Could you check a few things on this model? Use its own coordinates, in mm. A direction names the side the tool comes from. Coordinates: 2 decimals unless noted, no trailing zeros. Order: outer loops, then holes, each group sorted by start corner. A loop starts at its lowest first (then second) coordinate and runs counter-clockwise, first axis right, second up. Notation, with made-up numbers: (32, -9) - (38, -9) arc R6 ccw to (38, -2) - close; hole circle Ø9 at (-24, 39.5). An arc over 180 degrees is marked (long way). Answer as CSV lines item,"result". Start each with the question number.
1. I want a section at A-A, the plane x = 33. List the corners of the cut face in (y, z) for me, and give its area (3 significant figures).
2. I want a section at D-D, the plane y = -14.5. Count the separate pieces of the cut face and the enclosed holes in it, and give its area (3 significant figures).
3. I want a section at B-B, the plane z = -8.5. List the corners of the cut face in (x, y) for me.
4. I need wall thicknesses on probe 1 along X at (y, z) = (-12.7, -10); probe 2 along Y at (x, z) = (38.1, -8); probe 3 along X at (y, z) = (-14.75, -16.5). Which ranges of each line are inside material? Lowest first, please.
5. For faces 1 (the face through (25, -10, -2.108)), 2 (the face through (23, 0, -1)), 3 (the face through (48.692, -10, -13)), which set-ups out of +Z, -Z, +X, -X, +Y, -Y let a thin tool reach every point of the face, with its end or its side?
6. I want a section at C-C, the plane y = -3. List the corners of the cut face in (x, z) for me, and give its area (3 significant figures).
7. For pin 1 (6 mm diameter, centred on y = -19.5, z = -7, fed in from +X); pin 2 (5 mm diameter, centred on x = 44.5, y = -17.5, fed in from -Z); pin 3 (6 mm diameter, centred on x = 12.7, y = -12.7, fed in from +Z), each with a flat end and sliding along its axis, tell me the tip position at first contact or that it passes through.
8. Thinking about a two-plate mould opening in Y: for faces 4 (the face through (35.754, -13.673, -19.247)), 5 (the face through (25, -25.4, -13)), 6 (the face through (11.33, -10.56, -6.3)), 7 (the face through (25, -10, -23.292)), which applies, released by +Y, released by -Y, zero draft, split by the parting line, or undercut?
from build123d import *

# Parameters (mm, degrees)
SKETCH2_W           = 50.8
SKETCH2_H           = 25.4
BOSS_EXTRUDE2_DEPTH = 1.999996
SKETCH2_4_W         = 46.5836
SKETCH2_4_H         = 21.1836
BOSS_EXTRUDE3_DEPTH = 25.4
FILLET3_R           = 0.810638298
SKETCH3_R           = 2.54
CUT_EXTRUDE1_DEPTH  = 49.6918
SKETCH4_R           = 2.54
CUT_EXTRUDE2_DEPTH  = 24.2918


with BuildPart() as part:
    # Sketch2 → Boss-Extrude2 (new body)
    with BuildSketch(Plane(origin=(0, 0, 0), x_dir=(1, 0, 0), z_dir=(0, 1, 0))):
        with Locations((25.4, 12.7)):
            Rectangle(SKETCH2_W, SKETCH2_H)
    extrude(amount=BOSS_EXTRUDE2_DEPTH)

    # Sketch2<4> → Boss-Extrude3 (add)
    with BuildSketch(Plane(origin=(0, 0, 0), x_dir=(1, 0, 0), z_dir=(0, 1, 0))):
        with Locations((25.4, 12.7)):
            Rectangle(SKETCH2_4_W, SKETCH2_4_H)
    extrude(amount=-BOSS_EXTRUDE3_DEPTH)

    # Fillet3
    fillet3_edges = [part.edges().sort_by_distance(p)[0] for p in [
        (2.1082, -12.7, -2.1082),
        (2.1082, -12.7, -23.2918),
        (48.6918, -12.7, -23.2918),
        (48.6918, -12.7, -2.1082),
    ]]
    fillet(fillet3_edges, radius=FILLET3_R)

    # Sketch3 → Cut-Extrude1 (cut, through all)
    with BuildSketch(Plane(origin=(48.6918, 0, 0), x_dir=(0, 0, -1), z_dir=(1, 0, 0))):
        with Locations((12.7, -12.7)):
            Circle(SKETCH3_R)
    extrude(amount=-CUT_EXTRUDE1_DEPTH, mode=Mode.SUBTRACT)

    # Sketch4 → Cut-Extrude2 (cut, through all)
    with BuildSketch(Plane(origin=(0, 0, -23.2918), x_dir=(-1, 0, 0), z_dir=(0, 0, -1))):
        with Locations((-25.4, -12.7)):
            Circle(SKETCH4_R)
        with Locations((-38.1, -12.7)):
            Circle(SKETCH4_R)
        with Locations((-12.7, -12.7)):
            Circle(SKETCH4_R)
    extrude(amount=-CUT_EXTRUDE2_DEPTH, mode=Mode.SUBTRACT)


solid = part.part
Solved:
1,outline,"(-25.4, -23.29) - (0, -23.29) - (0, -25.4) - (2, -25.4) - (2, 0) - (0, 0) - (0, -2.11) - (-25.4, -2.11) - close; hole circle Ø5.08 at (-12.7, -12.7)"
1,area,"569 mm2"
2,separate pieces,"8"
2,enclosed holes,"0"
2,area,"630 mm2"
3,outline,"(0, 0) - (2.11, 0) - (2.11, -25.4) - (48.69, -25.4) - (48.69, 0) - (50.8, 0) - (50.8, 2) - (0, 2) - close; hole circle Ø5.08 at (12.7, -12.7); hole circle Ø5.08 at (25.4, -12.7); hole circle Ø5.08 at (38.1, -12.7)"
4,probe 1,"x = 2.11 to 10.16, 15.24 to 22.86, 27.94 to 35.56, 40.64 to 48.69"
4,probe 2,"y = -25.4 to -15.24, -10.16 to 2"
4,probe 3,"x = 2.11 to 11.2, 14.2 to 23.9, 26.9 to 36.6, 39.6 to 48.69"
5,face 1,"+Z, +X, -X, -Y"
5,face 2,"-Y"
5,face 3,"+Z, -Z, +X, -Y"
6,outline,"(2.11, -22.48) arc R0.81 ccw to (2.92, -23.29) - (47.88, -23.29) arc R0.81 ccw to (48.69, -22.48) - (48.69, -2.92) arc R0.81 ccw to (47.88, -2.11) - (2.92, -2.11) arc R0.81 ccw to (2.11, -2.92) - close"
6,area,"986 mm2"
7,pin 1,"stops at x = 48.69"
7,pin 2,"stops at z = -23.29"
7,pin 3,"stops at z = -2.11"
8,face 4,"undercut"
8,face 5,"released by -Y"
8,face 6,"undercut"
8,face 7,"zero draft"
